```python
from build123d import *

# Parameters (mm, degrees)
SKETCH_1_W          = 80
SKETCH_1_H          = 44
EXTRUDE_1_DEPTH     = 28
FILLET_1_R          = 13.5
FILLET_2_R          = 13.5
SKETCH_2_R          = 10
EXTRUDE_2_DEPTH     = 15
EXTRUDE_3_DEPTH     = 3.7
SKETCH_4_R          = 6.7
EXTRUDE_4_DEPTH     = 10
SKETCH_5_R          = 5.883118282
CUT_EXTRUDE_1_DEPTH = 20
FILLET_3_R          = 4
CUT_EXTRUDE_2_DEPTH = 8.5
EXTRUDE_5_DEPTH     = 14
FILLET_4_R          = 3
FILLET_5_R          = 3
SKETCH_9_R          = 1.5
CUT_EXTRUDE_3_DEPTH = 4


with BuildPart() as part:
    # Sketch 1 → Extrude 1 (new body)
    with BuildSketch(Plane.XY):
        Rectangle(SKETCH_1_W, SKETCH_1_H)
    extrude(amount=EXTRUDE_1_DEPTH)

    # Fillet 1
    fillet_1_edges = [part.edges().sort_by_distance(p)[0] for p in [
        (0, 22, 28),
    ]]
    fillet(fillet_1_edges, radius=FILLET_1_R)

    # Fillet 2
    fillet_2_edges = [part.edges().sort_by_distance(p)[0] for p in [
        (0, 22, 0),
    ]]
    fillet(fillet_2_edges, radius=FILLET_2_R)

    # Sketch 2 → Extrude 2 (add)
    with BuildSketch(Plane(origin=(40, 0, 0), x_dir=(0, 0, -1), z_dir=(1, 0, 0))):
        with Locations(Location((-13.5, 8.5, 0), (0, 0, 180))):
            Circle(SKETCH_2_R)
    extrude(amount=EXTRUDE_2_DEPTH)

    # Sketch 3 → Extrude 3 (add)
    with BuildSketch(Plane(origin=(55, 0, 0), x_dir=(0, 0, -1), z_dir=(1, 0, 0))):
        Polygon((-13.5, 18.5), (-22.160254038, 13.5), (-22.160254038, 3.5), (-13.5, -1.5), (-4.839745962, 3.5), (-4.839745962, 13.5), align=None)
    extrude(amount=EXTRUDE_3_DEPTH)

    # Sketch 4 → Extrude 4 (add)
    with BuildSketch(Plane(origin=(58.7, 0, 0), x_dir=(0, 0, -1), z_dir=(1, 0, 0))):
        with Locations((-13.5, 8.5)):
            Circle(SKETCH_4_R)
    extrude(amount=EXTRUDE_4_DEPTH)

    # Sketch 5 → Cut-Extrude 1 (cut)
    with BuildSketch(Plane(origin=(68.7, 0, 0), x_dir=(0, 0, -1), z_dir=(1, 0, 0))):
        with Locations((-13.5, 8.5)):
            Circle(SKETCH_5_R)
    extrude(amount=-CUT_EXTRUDE_1_DEPTH, mode=Mode.SUBTRACT)

    # Fillet 3
    fillet_3_edges = [part.edges().sort_by_distance(p)[0] for p in [
        (40, -6.75, 0),
        (40, 18.045941546, 24.045941546),
        (-40, -6.75, 0),
        (-40, 18.045941546, 3.954058454),
        (-40, 22, 14),
        (-40, 18.045941546, 24.045941546),
        (40, -6.75, 28),
        (-40, -6.75, 28),
    ]]
    fillet(fillet_3_edges, radius=FILLET_3_R)

    # Sketch 7 → Cut-Extrude 2 (cut)
    with BuildSketch(Plane.XZ.offset(22)):
        with BuildLine():
            Line((-36, 2), (36, 2))
            ThreePointArc((36, 2), (37.414213562, 2.585786438), (38, 4))
            Line((38, 4), (38, 24))
            ThreePointArc((38, 24), (37.414213562, 25.414213562), (36, 26))
            Line((36, 26), (-36, 26))
            ThreePointArc((-36, 26), (-37.414213562, 25.414213562), (-38, 24))
            Line((-38, 24), (-38, 4))
            ThreePointArc((-38, 4), (-37.414213562, 2.585786438), (-36, 2))
        make_face()
    extrude(amount=-CUT_EXTRUDE_2_DEPTH, mode=Mode.SUBTRACT)

    # Sketch 8 → Extrude 5 (add)
    with BuildSketch(Plane.XZ.offset(13.5)):
        Polygon((-18, 16), (-18, 20), (18, 20), (18, 16), (22.5, 16), (22.5, 12), (18, 12), (18, 8), (-18, 8), (-18, 12), (-22.5, 12), (-22.5, 16), align=None)
    extrude(amount=EXTRUDE_5_DEPTH)

    # Fillet 4
    fillet_4_edges = [part.edges().sort_by_distance(p)[0] for p in [
        (0, -27.5, 20),
    ]]
    fillet(fillet_4_edges, radius=FILLET_4_R)

    # Fillet 5
    fillet_5_edges = [part.edges().sort_by_distance(p)[0] for p in [
        (0, -27.5, 8),
    ]]
    fillet(fillet_5_edges, radius=FILLET_5_R)

    # Sketch 9 → Cut-Extrude 3 (cut)
    with BuildSketch(Plane.XZ.offset(13.5)):
        with Locations(Location((-24.3, 20, 0), (0, 0, 270))):
            Circle(SKETCH_9_R)
        with Locations(Location((-18.9, 20, 0), (0, 0, 270))):
            Circle(SKETCH_9_R)
        with Locations(Location((-13.5, 20, 0), (0, 0, 270))):
            Circle(SKETCH_9_R)
        with Locations(Location((-8.1, 20, 0), (0, 0, 270))):
            Circle(SKETCH_9_R)
        with Locations(Location((-2.7, 20, 0), (0, 0, 270))):
            Circle(SKETCH_9_R)
        with Locations(Location((2.7, 20, 0), (0, 0, 270))):
            Circle(SKETCH_9_R)
        with Locations(Location((8.1, 20, 0), (0, 0, 270))):
            Circle(SKETCH_9_R)
        with Locations(Location((13.5, 20, 0), (0, 0, 270))):
            Circle(SKETCH_9_R)
        with Locations(Location((18.9, 20, 0), (0, 0, 270))):
            Circle(SKETCH_9_R)
        with Locations(Location((24.3, 20, 0), (0, 0, 270))):
            Circle(SKETCH_9_R)
        with Locations(Location((-24.3, 8, 0), (0, 0, 270))):
            Circle(SKETCH_9_R)
        with Locations(Location((-18.9, 8, 0), (0, 0, 270))):
            Circle(SKETCH_9_R)
        with Locations(Location((-13.5, 8, 0), (0, 0, 270))):
            Circle(SKETCH_9_R)
        with Locations(Location((-8.1, 8, 0), (0, 0, 270))):
            Circle(SKETCH_9_R)
        with Locations(Location((-2.7, 8, 0), (0, 0, 270))):
            Circle(SKETCH_9_R)
        with Locations(Location((2.7, 8, 0), (0, 0, 270))):
            Circle(SKETCH_9_R)
        with Locations(Location((8.1, 8, 0), (0, 0, 270))):
            Circle(SKETCH_9_R)
        with Locations(Location((13.5, 8, 0), (0, 0, 270))):
            Circle(SKETCH_9_R)
        with Locations(Location((18.9, 8, 0), (0, 0, 270))):
            Circle(SKETCH_9_R)
        with Locations(Location((24.3, 8, 0), (0, 0, 270))):
            Circle(SKETCH_9_R)
    extrude(amount=-CUT_EXTRUDE_3_DEPTH, mode=Mode.SUBTRACT)


solid = part.part
```
Model file for the job. Use its own axes, mm. A direction names the side the tool comes from. Give positions to 0.01 mm unless a question says otherwise; leave off trailing zeros. Loops run counter-clockwise (first coordinate to the right, second up) from the corner with the lowest first, then second, coordinate; pieces in that order, holes last. Notation, with made-up numbers: (55.5, 31) -> (81.5, 31) arc R15 ccw to (81.5, 60) -> close; hole circle Ø6 at (52.5, -15.75). An arc over 180 degrees is marked (long way). Use CSV: the item, a comma, the result in double quotes. Start each with the question number.
1) Slice it at A-A on y = -18. Give the cut face in (x, z), plus the area to 3 significant figures.
2) Mould opens along Y. For faces 1 (the cylindrical face through (24.37, -11.53, 21.5)), 2 (the flat face through (-13, -9.5, 20)), 3 (the flat face through (-3, -9.5, 20)), 4 (the cylindrical face through (0.52, 18.15, 4.06)) say: released by +Y, released by -Y, zero draft, split by the parting line, or undercut.
3) Slice it at C-C on x = 27. Give the cut face in (y, z), plus the area to 3 significant figures.
4) Tool access for faces 5 (the cylindrical face through (47.4, 5.5, 23.04)), 6 (the flat face through (14, -9.5, 8)), 7 (the flat face through (-20, -20, 16)): list every direction of +Z, -Z, +X, -X, +Y, -Y with a clear straight run to the whole face (end or side of a thin tool).
5) Wall check: line 1 (X direction, y = -21, z = 11.25); line 2 (Z direction, x = -8.1, y = -12); line 3 (Z direction, x = 18, y = -12). Give the ranges that are in metal, low to high.
6) Flat gauge pins, fed straight in: pin 1 Ø12 at (x, y) = (53.5, -1.5) entering from +Z; pin 2 Ø0.9 at (x, z) = (24.5, 8) entering from -Y; pin 3 Ø6 at (y, z) = (-11.5, 9.5) entering from +X; pin 4 Ø10 at (y, z) = (14, 3.5) entering from +X. Where does each tip first touch, or does it go through?
7) Slice it at D-D on x = 13.5. Give the cut face in (y, z), plus the area to 3 significant figures.
8) Slice it at B-B on x = -24.3. Give the cut face in (y, z).
Computed values:
1,outline,"(-40, 4) arc R4 ccw to (-36, 0) -> (36, 0) arc R4 ccw to (40, 4) -> (40, 24) arc R4 ccw to (36, 28) -> (-36, 28) arc R4 ccw to (-40, 24) -> close; (-22.5, 12) -> (-18, 12) -> (-18, 8) -> (18, 8) -> (18, 12) -> (22.5, 12) -> (22.5, 16) -> (18, 16) -> (18, 20) -> (-18, 20) -> (-18, 16) -> (-22.5, 16) -> close; hole (-38, 4) arc R2 ccw to (-36, 2) -> (36, 2) arc R2 ccw to (38, 4) -> (38, 24) arc R2 ccw to (36, 26) -> (-36, 26) arc R2 ccw to (-38, 24) -> close"
1,area,"874 mm^2"
2,face 1,"zero draft"
2,face 2,"undercut"
2,face 3,"undercut"
2,face 4,"released by +Y"
3,outline,"(-22, 0) -> (8.5, 0) arc R13.5 ccw to (22, 13.5) -> (22, 14.5) arc R13.5 ccw to (8.5, 28) -> (-22, 28) -> (-22, 26) -> (-13.5, 26) -> (-13.5, 2) -> (-22, 2) -> close"
3,area,"950 mm^2"
4,face 5,"+X"
4,face 6,"none"
4,face 7,"-Y"
5,line 1,"x = -40 to -38, -18 to 18, 38 to 40"
5,line 2,"z = 0 to 6.5, 9.5 to 18.5, 21.5 to 28"
5,line 3,"z = 0 to 6.8, 9.2 to 18.8, 21.2 to 28"
6,pin 1,"stops at z = 22.67"
6,pin 2,"stops at y = -9.5"
6,pin 3,"stops at x = 40"
6,pin 4,"stops at x = 68.7"
7,outline,"(-27.5, 11) arc R3 ccw to (-24.5, 8) -> (-13.5, 8) -> (-13.5, 9.5) -> (-9.5, 9.5) -> (-9.5, 6.5) -> (-13.5, 6.5) -> (-13.5, 2) -> (-22, 2) -> (-22, 0) -> (8.5, 0) arc R13.5 ccw to (22, 13.5) -> (22, 14.5) arc R13.5 ccw to (8.5, 28) -> (-22, 28) -> (-22, 26) -> (-13.5, 26) -> (-13.5, 21.5) -> (-9.5, 21.5) -> (-9.5, 18.5) -> (-13.5, 18.5) -> (-13.5, 20) -> (-24.5, 20) arc R3 ccw to (-27.5, 17) -> close"
7,area,"1,090 mm^2"
8,outline,"(-22, 0) -> (8.5, 0) arc R13.5 ccw to (22, 13.5) -> (22, 14.5) arc R13.5 ccw to (8.5, 28) -> (-22, 28) -> (-22, 26) -> (-13.5, 26) -> (-13.5, 21.5) -> (-9.5, 21.5) -> (-9.5, 18.5) -> (-13.5, 18.5) -> (-13.5, 9.5) -> (-9.5, 9.5) -> (-9.5, 6.5) -> (-13.5, 6.5) -> (-13.5, 2) -> (-22, 2) -> close"
